```python
from build123d import *

# Parameters (mm, degrees)
F1_DEPTH = 20
F2_R     = 1.25
F3_DEPTH = 6
F5_R     = 2.75
F6_DEPTH = 5


with BuildPart() as f1:
    # F0 (on Top) → F1 (new body)
    with BuildSketch(Plane.XY):
        with BuildLine():
            Line((-9.25, -9), (9.25, -9))
            Line((9.25, -9), (9.25, 1.95))
            ThreePointArc((9.25, 1.95), (8.3891203434, 5.8383820078), (5.9673854088, 9))
            ThreePointArc((5.9673854088, 9), (4.1312205072, 9.0265556821), (4.25, 7.1940442409))
            ThreePointArc((4.25, 7.1940442409), (0, -4.8), (-4.25, 7.1940442409))
            ThreePointArc((-4.25, 7.1940442409), (-4.0659177332, 8.9522005817), (-5.8240740741, 9.1362828486))
            ThreePointArc((-5.8240740741, 9.1362828486), (-8.3497061381, 5.9305662169), (-9.25, 1.95))
            Line((-9.25, 1.95), (-9.25, -9))
        make_face()
    extrude(amount=F1_DEPTH)

    # F2 (on face) → F3 (cut)
    with BuildSketch(Plane.XZ.offset(9)):
        with Locations((0, 14.75)):
            Circle(F2_R)
        with Locations((0, 5.25)):
            Circle(F2_R)
    extrude(amount=-F3_DEPTH, mode=Mode.SUBTRACT)

    # F5 (on offset) → F6 (cut)
    with BuildSketch(Plane.XZ.offset(6.8)):
        with Locations((0, 14.75)):
            Circle(F5_R)
        with Locations((0, 5.25)):
            Circle(F5_R)
    extrude(amount=-F6_DEPTH, mode=Mode.SUBTRACT)


solid = f1.part
```
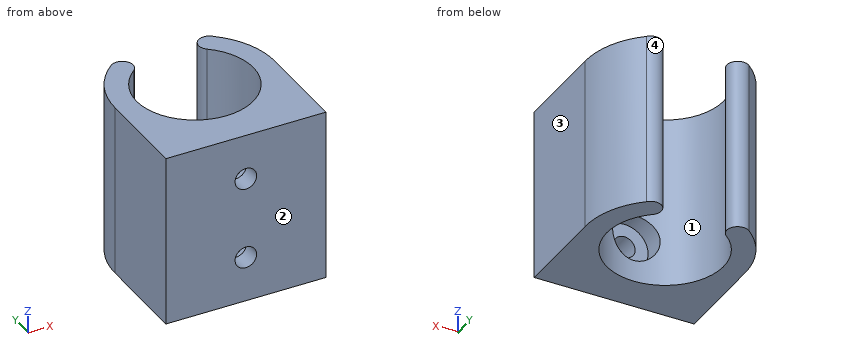
Geometry check sheet. Reference: the model listing, model coordinates, mm. Face numbers are marked on the shaded views. Coordinates: 2 decimals unless noted, no trailing zeros. Loops run counter-clockwise (first coordinate to the right, second up) from the corner with the lowest first, then second, coordinate; pieces in that order, holes last.
Item 1: Sectioned sample at C-C, the plane y = -2.75. Record the boundary of the cut face in (x, z).
Item 2: Go/stop test with flat-tipped pins: pin 1 Ø6 at (x, z) = (0, 5) entering from +Y; pin 2 Ø1.5 at (y, z) = (6, 17.5) entering from -X; pin 3 Ø5 at (x, z) = (1.5, 10) entering from +Y. Record where each tip stops, or that it passes through.
Item 3: Sectioned sample at B-B, the plane x = 0. Record the boundary of the cut face in (y, z), then the cut area to 3 significant figures.
Item 4: Release check for a two-part mould opening along X. For the marked faces 1, 2, 3 and 4 record: released by +X, released by -X, zero draft, split by the parting line, or undercut.
Item 5: Sectioned sample at D-D, the plane z = 18. Record the boundary of the cut face in (x, y).
Item 6: Thickness scan on line 1 (Z direction, x = 0, y = -7.3); line 2 (X direction, y = -5.15, z = 5.25); line 3 (X direction, y = 1.95, z = 4.5). Record the ranges inside material, lowest first.
Item 7: Sectioned sample at A-A, the plane z = 14.75. Record the boundary of the cut face in (x, y).
Check result:
1. outline: (-9.25, 0) - (-4.84, 0) - (-4.84, 20) - (-9.25, 20) - close; (4.84, 0) - (9.25, 0) - (9.25, 20) - (4.84, 20) - close
2. pin 1: stops at y = -4.1
2. pin 2: stops at x = -8.64
2. pin 3: stops at y = 8.86
3. outline: (-9, 0) - (-4.8, 0) - (-4.8, 2.5) - (-6.8, 2.5) - (-6.8, 4) - (-9, 4) - close; (-9, 6.5) - (-6.8, 6.5) - (-6.8, 8) - (-4.8, 8) - (-4.8, 12) - (-6.8, 12) - (-6.8, 13.5) - (-9, 13.5) - close; (-9, 16) - (-6.8, 16) - (-6.8, 17.5) - (-4.8, 17.5) - (-4.8, 20) - (-9, 20) - close
3. area: 51.0 mm2
4. face 1: undercut
4. face 2: zero draft
4. face 3: released by +X
4. face 4: undercut
5. outline: (-9.25, -9) - (9.25, -9) - (9.25, 1.95) arc R9.21 ccw to (5.97, 9) arc R1.25 ccw (long way) to (4.25, 7.19) arc R6.75 cw (long way) to (-4.25, 7.19) arc R1.25 ccw to (-5.82, 9.14) arc R9.25 ccw to (-9.25, 1.95) - close
6. line 1: z = 0 to 4, 6.5 to 13.5, 16 to 20
6. line 2: x = -9.25 to -2.75, 2.75 to 9.25
6. line 3: x = -9.25 to -6.75, 6.75 to 9.25
7. outline: (-9.25, -9) - (-1.25, -9) - (-1.25, -6.8) - (-2.75, -6.8) - (-2.75, -4.21) arc R6.75 cw to (-4.25, 7.19) arc R1.25 ccw to (-5.82, 9.14) arc R9.25 ccw to (-9.25, 1.95) - close; (1.25, -9) - (9.25, -9) - (9.25, 1.95) arc R9.21 ccw to (5.97, 9) arc R1.25 ccw (long way) to (4.25, 7.19) arc R6.75 cw to (2.75, -4.21) - (2.75, -6.8) - (1.25, -6.8) - close
